Geometry check sheet. Reference: the model listing, model coordinates, mm. A direction names the side the tool comes from. Coordinates: 2 decimals unless noted, no trailing zeros. Order: outer loops, then holes, each group sorted by start corner. A loop starts at its lowest first (then second) coordinate and runs counter-clockwise, first axis right, second up. Notation, with made-up numbers: (10.25, 20) - (48.25, 20) arc R12 ccw to (48.25, 34) - close; hole circle Ø5 at (66.25, 37.5). An arc over 180 degrees is marked (long way). Return JSON: item names as keys, results as strings. Group by question number.
Item 1: Tool access check on faces 1 (the flat face through (6, -31.137, 42)), 2 (the flat face through (0, -39, 19)). Record the directions out of +Z, -Z, +X, -X, +Y, -Y that give a thin tool (end or side, any length) a straight path to the whole face; none if there is none.
Item 2: Section check B-B on x = 7. Enter the section's corners in (y, z), then the cut area to 3 significant figures.
Item 3: Scan lines: probe 1 along Z at (x, y) = (21.5, -27.25); probe 2 along Y at (x, z) = (7, 5.5). Record each from-to range of solid material in increasing order.
Item 4: Draft check along Y on faces 3 (the cylindrical face through (28.121, -45.216, 6.439)), 4 (the flat face through (28, -51.854, 6)), 5 (the cylindrical face through (38.92, -43.29, 6.44)), 6 (the flat face through (28, -26.454, 6)). Enter one of: pulls with the +Y half, pulls with the -Y half, needs draft (parallel to the pull), parting line crosses it, or undercut.
Item 5: Section check D-D on x = 20.5. Enter the section's corners in (y, z).
Item 6: Section check C-C on z = 6.5. Enter the section's corners in (x, y).
Item 7: Section check A-A on y = -41.5. Enter the section's corners in (x, z), then the cut area to 3 significant figures.
Item 8: Gauge pin test, flat ends, axial feed: pin 1 (5 mm diameter, centred on x = 49, y = -49, fed in from +Z); pin 2 (1 mm diameter, centred on y = -34, z = 27.5, fed in from +X); pin 3 (1.5 mm diameter, centred on x = 8.5, z = 14, fed in from -Y). Record the tip position at first contact, or that the pin passes through.
from build123d import *

# Parameters (mm, degrees)
F0_W     = 25.4
F0_H     = 38.1
F1_DEPTH = 12.7
F2_W     = 31.75
F2_H     = 25.4
F3_DEPTH = 12.7
F5_DEPTH = 12.7
F6_R     = 6.832964
F6_R_2   = 6.803231
F7_DEPTH = 12.7


with BuildPart() as f1:
    # F0 (on Right) → F1 (new body)
    with BuildSketch(Plane.YZ):
        with Locations((-38.928264, 19.05)):
            Rectangle(F0_W, F0_H)
        with BuildLine():
            ThreePointArc((-26.228264, 38.1), (-38.928264, 50.8), (-51.628264, 38.1))
            Line((-51.628264, 38.1), (-26.228264, 38.1))
        make_face()
    extrude(amount=F1_DEPTH)

    # F2 (on Top) → F3 (join)
    with BuildSketch(Plane.XY):
        with BuildLine():
            ThreePointArc((44.319397, -51.85383), (57.019397, -39.15383), (44.319397, -26.45383))
            Line((44.319397, -26.45383), (44.319397, -51.85383))
        make_face()
        with Locations((28.444397, -39.15383)):
            Rectangle(F2_W, F2_H)
    extrude(amount=F3_DEPTH)

    # F4 (on face) → F5 (cut)
    with BuildSketch(Plane.YZ.offset(12.7)):
        with BuildLine():
            ThreePointArc((-31.137236, 48.129451), (-39.756961, 56.367), (-47.595407, 47.382814))
            ThreePointArc((-47.595407, 47.382814), (-39.503817, 50.786951), (-31.137236, 48.129451))
        make_face()
        with BuildLine():
            ThreePointArc((-31.137236, 48.129451), (-39.503817, 50.786951), (-47.595407, 47.382814))
            Line((-47.595407, 47.382814), (-47.595407, 34.682814))
            ThreePointArc((-47.595407, 34.682814), (-39.009555, 27.191903), (-31.137236, 35.429451))
            Line((-31.137236, 35.429451), (-31.137236, 48.129451))
        make_face()
    extrude(amount=-F5_DEPTH, mode=Mode.SUBTRACT)

    # F6 (on face) → F7 (cut)
    with BuildSketch(Plane.XY.offset(12.7)):
        with Locations((24.967661, -39.15383)):
            Circle(F6_R)
        with Locations((44.319397, -39.15383)):
            Circle(F6_R_2)
    extrude(amount=-F7_DEPTH, mode=Mode.SUBTRACT)


solid = f1.part
Computed:
{
 "1": {"face 1": "+Z, +X, -X", "face 2": "+Z, -Z, -X, +Y, -Y"},
 "2": {"outline": "(-51.63, 0) - (-26.23, 0) - (-26.23, 38.1) arc R12.7 ccw to (-31.14, 48.13) - (-31.14, 35.43) arc R8.25 cw to (-47.6, 34.68) - (-47.6, 47.38) arc R12.7 ccw to (-51.63, 38.1) - close", "area": "877 mm²"},
 "3": {"probe 1": "z = 0 to 12.7", "probe 2": "y = -51.63 to -26.23"},
 "4": {"face 3": "undercut", "face 4": "pulls with the -Y half", "face 5": "undercut", "face 6": "pulls with the +Y half"},
 "5": {"outline": "(-51.85, 0) - (-44.32, 0) - (-44.32, 12.7) - (-51.85, 12.7) - close; (-33.98, 0) - (-26.45, 0) - (-26.45, 12.7) - (-33.98, 12.7) - close"},
 "6": {"outline": "(0, -51.63) - (12.57, -51.63) - (12.57, -51.85) - (44.32, -51.85) arc R12.7 ccw to (44.32, -26.45) - (12.7, -26.45) - (12.7, -26.23) - (0, -26.23) - close; hole circle Ø13.67 at (24.97, -39.15); hole circle Ø13.61 at (44.32, -39.15)"},
 "7": {"outline": "(0, 0) - (18.55, 0) - (18.55, 12.7) - (12.7, 12.7) - (12.7, 27.46) - (0, 27.46) - close; (31.39, 0) - (37.93, 0) - (37.93, 12.7) - (31.39, 12.7) - close; (50.71, 0) - (56.8, 0) - (56.8, 12.7) - (50.71, 12.7) - close", "area": "584 mm²"},
 "8": {"pin 1": "stops at z = 12.7", "pin 2": "stops at x = 12.7", "pin 3": "stops at y = -51.63"}
}
